Work out the finished part from the listing and answer in its coordinate system (mm). A direction names the side the tool comes from. Give positions to 0.01 mm unless a question says otherwise; leave off trailing zeros. Order: outer loops, then holes, each group sorted by start corner. A loop starts at its lowest first (then second) coordinate and runs counter-clockwise, first axis right, second up. Notation, with made-up numbers: (-39.5, 80) - (-26.5, 80) arc R16 ccw to (-26.5, 85) - close; hole circle Ø6 at (82.5, 33.5). An arc over 180 degrees is marked (long way). Put each result on its own line as item: value.
```python
from build123d import *

# Parameters (mm, degrees)
F0_W          = 4.9083643031
F0_H          = 38.6046577501
F1_DEPTH      = 25.4
F3_W          = 4.1379593313
F3_H          = 22.0691054128
F4_DEPTH      = 8.89
F4_DEPTH_BACK = 25.4
F5_W          = 4.6289921738
F5_H          = 21.6983995633
F6_DEPTH      = 17.78


with BuildPart() as f1:
    # F0 (on Front) → F1 (new body)
    with BuildSketch(Plane.XZ):
        Polygon((5.08, 0), (0, 0), (-16.51, -19.302328875), (21.59, -19.302328875), (21.59, 19.302328875), align=None)
        with Locations((24.0441821516, 0)):
            Rectangle(F0_W, F0_H)
        Polygon((26.4983643031, 19.302328875), (26.4983643031, -19.302328875), (64.5983643031, -19.302328875), (48.0883643031, 0), (43.0083643031, 0), align=None)
    extrude(amount=F1_DEPTH)

    # F3 (on offset) → F4 (cut, two sides)
    with BuildSketch(Plane.XY.offset(11.684)) as f4_sk:
        with Locations((18.0260073394, -12.533511268)):
            Rectangle(F3_W, F3_H)
    extrude(amount=-F4_DEPTH, mode=Mode.SUBTRACT)
    extrude(f4_sk.sketch, amount=F4_DEPTH_BACK, mode=Mode.SUBTRACT)

    # F5 (on offset) → F6 (cut)
    with BuildSketch(Plane.XY.offset(11.684)):
        with Locations((9.8292285111, -12.3650435708)):
            Rectangle(F5_W, F5_H)
    extrude(amount=-F6_DEPTH, mode=Mode.SUBTRACT)


solid = f1.part
```
(1) Straight lines are drawn through the part: line 1 (Y direction, x = 16, z = 10); line 2 (X direction, y = -17, z = 11); line 3 (X direction, y = -16, z = 9.5). For each, find the intervals that lie inside material, in ascending order.
Geometry check:
line 1: y = -25.4 to -23.57, -1.5 to 0
line 2: x = 14.49 to 15.96, 20.09 to 33.6
line 3: x = 13.21 to 15.96, 20.09 to 34.88
(2) Determine the mould class of faces 1 (the face through (34.869, -12.522, 9.516)), 2 (the face through (23, -25.4, -4)), 3 (the face through (18, -1.499, 8)) for opening direction X: pulls with the +X half, pulls with the -X half, needs draft (parallel to the pull), parting line crosses it, or undercut.
Geometry check:
face 1: pulls with the +X half
face 2: needs draft
face 3: undercut
(3) Section B-B, the plane z = -1 is taken. Write down the section's boundary in (x, y), then the cut area to 3 significant figures.
Geometry check:
outline: (-0.86, -25.4) - (48.94, -25.4) - (48.94, 0) - (-0.86, 0) - close; hole (7.51, -23.21) - (12.14, -23.21) - (12.14, -1.52) - (7.51, -1.52) - close
area: 1,160 mm²
(4) Section C-C, the plane x = 50.5 is taken. Write down the section's boundary in (y, z), then the cut area to 3 significant figures.
Geometry check:
outline: (-25.4, -19.3) - (0, -19.3) - (0, -2.82) - (-25.4, -2.82) - close
area: 419 mm²
(5) Section A-A, the plane y = -13.5 is taken. Write down the section's boundary in (x, z), then the cut area to 3 significant figures.
Geometry check:
outline: (-16.51, -19.3) - (64.6, -19.3) - (48.09, 0) - (43.01, 0) - (26.5, 19.3) - (21.59, 19.3) - (20.09, 17.55) - (20.09, 2.79) - (15.96, 2.79) - (15.96, 12.72) - (12.14, 8.26) - (12.14, -6.1) - (7.51, -6.1) - (7.51, 2.85) - (5.08, 0) - (0, 0) - close
area: 1,560 mm²
(6) Given pin 1 (2 mm diameter, centred on y = -19.5, z = -7, fed in from -X); pin 2 (1.4 mm diameter, centred on x = 11, y = -8, fed in from +Z); pin 3 (1.5 mm diameter, centred on x = 1.5, y = -16, fed in from +Z); pin 4 (12 mm diameter, centred on x = -4.5, z = 8, fed in from +Y), each flat-ended and moving along its own axis, determine where each tip first touches the part or whether it passes through.
Geometry check:
pin 1: stops at x = -6.84
pin 2: stops at z = -6.1
pin 3: stops at z = 0
pin 4: passes through
(7) Section D-D, the plane z = -9.5 is taken. Write down the section's boundary in (x, y), then the cut area to 3 significant figures.
Geometry check:
outline: (-8.13, -25.4) - (56.21, -25.4) - (56.21, 0) - (-8.13, 0) - close
area: 1,630 mm²
(8) A tool of negligible diameter and unlimited length cuts with its end or side. For faces 4 (the face through (46, -13, 0)), 5 (the face through (3, -13, 0)), 6 (the face through (18, -12, 2.794)), from which of +Z, -Z, +X, -X, +Y, -Y can it reach the whole face along a straight path? Write none if from no direction.
Geometry check:
face 4: +Z, +X, +Y, -Y
face 5: +Z, -X, +Y, -Y
face 6: +Z
